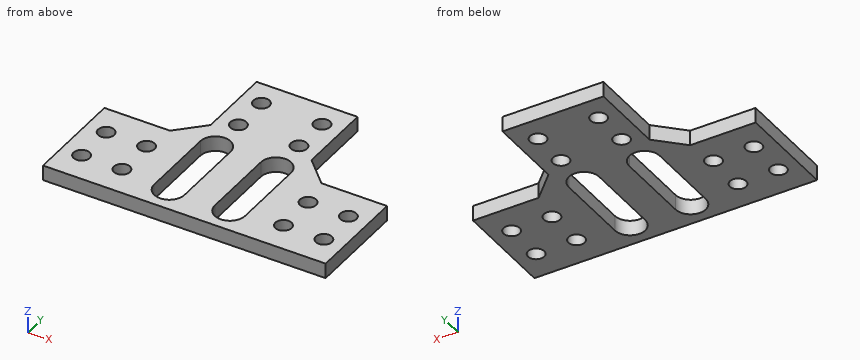
```python
from build123d import *

# Parameters (mm, degrees)
EXTRUDE_1_DEPTH     = 3
SKETCH_2_R          = 1.6
CUT_EXTRUDE_1_DEPTH = 3
CUT_EXTRUDE_2_DEPTH = 10


with BuildPart() as part:
    # 草图1 → 凸台-拉伸1 (new body)
    with BuildSketch(Plane.XY):
        Polygon((0, 0), (56, 0), (56, 20), (43, 20), (38, 25), (38, 40), (18, 40), (18, 25), (13, 20), (0, 20), align=None)
    extrude(amount=EXTRUDE_1_DEPTH)

    # 草图2 → 切除-拉伸1 (cut)
    with BuildSketch(Plane.XY.offset(3)):
        with Locations((22, 35)):
            Circle(SKETCH_2_R)
        with Locations((34, 35)):
            Circle(SKETCH_2_R)
        with Locations((22, 27.5)):
            Circle(SKETCH_2_R)
        with Locations((34, 27.5)):
            Circle(SKETCH_2_R)
        with Locations((4, 14)):
            Circle(SKETCH_2_R)
        with Locations((4, 6)):
            Circle(SKETCH_2_R)
        with Locations((12, 14)):
            Circle(SKETCH_2_R)
        with Locations((12, 6)):
            Circle(SKETCH_2_R)
        with Locations((52, 14)):
            Circle(SKETCH_2_R)
        with Locations((52, 6)):
            Circle(SKETCH_2_R)
        with Locations((44, 6)):
            Circle(SKETCH_2_R)
        with Locations((44, 14)):
            Circle(SKETCH_2_R)
    extrude(amount=-CUT_EXTRUDE_1_DEPTH, mode=Mode.SUBTRACT)

    # 草图3 → 切除-拉伸2 (cut)
    with BuildSketch(Plane.XY.offset(3)):
        with BuildLine():
            Line((25, 20), (25, 5))
            ThreePointArc((25, 5), (22, 2), (19, 5))
            Line((19, 5), (19, 20))
            ThreePointArc((19, 20), (22, 23), (25, 20))
        make_face()
        with BuildLine():
            Line((37, 20), (37, 5))
            ThreePointArc((37, 5), (34, 2), (31, 5))
            Line((31, 5), (31, 20))
            ThreePointArc((31, 20), (34, 23), (37, 20))
        make_face()
    extrude(amount=-CUT_EXTRUDE_2_DEPTH, mode=Mode.SUBTRACT)


solid = part.part
```
Here's how the part is built. I have some questions about the finished solid (model axes, mm). Give positions to 0.01 mm unless a question says otherwise; leave off trailing zeros. Loops run counter-clockwise (first coordinate to the right, second up) from the corner with the lowest first, then second, coordinate; pieces in that order, holes last. Notation, with made-up numbers: (45, -21) -> (61, -21) arc R24 cw to (61, 4) -> close; hole circle Ø2 at (33.5, 40.5). An arc over 180 degrees is marked (long way). Use one line per item in the form item = value. Start each with the question number.
1) Imagine slicing it at A-A (y = 6). Please give me the cut outline in (x, z), then the cut area to 3 significant figures.
2) Imagine slicing it at D-D (y = 27.5). Please give me the cut outline in (x, z).
3) For P1, Ø0.9, axis at y = 31.5, z = 1.5, coming from the +X side, with a flat end and sliding along its axis, tell me the tip position at first contact or that it passes through.
4) Please list where these lines run through material, in increasing order: line 1 along X through (y, z) = (16, 1.4); line 2 along Y through (x, z) = (44, 1.25); line 3 along Y through (x, z) = (22, 1.55).
5) Imagine slicing it at C-C (z = 1.65). Count the separate pieces of the cut face and the enclosed holes in it, then the cut area to 3 significant figures.
6) Imagine slicing it at B-B (x = 52). Please give me the cut outline in (y, z).
Check values:
q1.outline = (0, 0) -> (2.4, 0) -> (2.4, 3) -> (0, 3) -> close; (5.6, 0) -> (10.4, 0) -> (10.4, 3) -> (5.6, 3) -> close; (13.6, 0) -> (19, 0) -> (19, 3) -> (13.6, 3) -> close; (25, 0) -> (31, 0) -> (31, 3) -> (25, 3) -> close; (37, 0) -> (42.4, 0) -> (42.4, 3) -> (37, 3) -> close; (45.6, 0) -> (50.4, 0) -> (50.4, 3) -> (45.6, 3) -> close; (53.6, 0) -> (56, 0) -> (56, 3) -> (53.6, 3) -> close
q1.area = 93.6 mm^2
q2.outline = (18, 0) -> (20.4, 0) -> (20.4, 3) -> (18, 3) -> close; (23.6, 0) -> (32.4, 0) -> (32.4, 3) -> (23.6, 3) -> close; (35.6, 0) -> (38, 0) -> (38, 3) -> (35.6, 3) -> close
q3.P1 = 38
q4.line_1 = 0 to 19, 25 to 31, 37 to 56
q4.line_2 = 0 to 4.4, 7.6 to 12.4, 15.6 to 20
q4.line_3 = 0 to 2, 23 to 25.9, 29.1 to 33.4, 36.6 to 40
q5.separate_pieces = 1
q5.enclosed_holes = 14
q5.area = 1,210 mm^2
q6.outline = (0, 0) -> (4.4, 0) -> (4.4, 3) -> (0, 3) -> close; (7.6, 0) -> (12.4, 0) -> (12.4, 3) -> (7.6, 3) -> close; (15.6, 0) -> (20, 0) -> (20, 3) -> (15.6, 3) -> close
